Verification items for the finished model (mm, model axes). Face numbers are marked on the shaded views. A direction names the side the tool comes from. Coordinates: 2 decimals unless noted, no trailing zeros. Loops run counter-clockwise (first coordinate to the right, second up) from the corner with the lowest first, then second, coordinate; pieces in that order, holes last. Notation, with made-up numbers: (88.5, 77) -> (95.5, 77) arc R18 cw to (95.5, 90) -> close; hole circle Ø1 at (12.5, 53.5). An arc over 180 degrees is marked (long way). Answer as a JSON object with one key per item and string values. Group by question number.
Q1. Gauge pin test, flat ends, axial feed: pin 1 Ø2 at (x, z) = (2, -1) entering from +Y; pin 2 Ø1 at (x, y) = (7.5, 0.5) entering from +Z; pin 3 Ø1.5 at (x, y) = (12, -1.5) entering from +Z. Record the tip position at first contact, or that the pin passes through.
Q2. Cross-section at B-B on z = 0. Record the boundary of the cut face in (x, y), and give its area (3 significant figures).
Q3. Set-up check for the marked faces 1 and 2: record each of +Z, -Z, +X, -X, +Y, -Y from which the full face is reachable in a straight line by a thin tool's end or side.
Q4. Cross-section at A-A on y = 0. Record the boundary of the cut face in (x, z).
Q5. Scan lines: L1, parallel to X at y = -1.05, z = -1.3; L2, parallel to X at y = 1.7, z = 0; L3, parallel to Z at x = 7.5, y = 0.15. Record each from-to range of solid material in increasing order.
Q6. Cross-section at C-C on x = 5.5. Record the boundary of the cut face in (y, z), and give its area (3 significant figures).
```python
from build123d import *

# Parameters (mm, degrees)
CHAMFER1_SIZE       = 0.1
FILLET1_R           = 0.16
EXTRUDE1_DEPTH      = 15.059160715
EXTRUDE1_DEPTH_BACK = 15.059160715
SKETCH2_W           = 0.2
SKETCH2_H           = 0.2


with BuildPart() as part:
    # Sketch1 → Revolve1 (revolve)
    with BuildSketch(Plane.XY, mode=Mode.PRIVATE) as revolve1_sk:
        Polygon((0, 1.9), (0, 0), (13.8, 0), (13.8, 1), (1.3, 1), (1.3, 1.9), align=None)
    revolve(revolve1_sk.sketch.rotate(Axis((0, 0, 0), (1, 0, 0)), 90), axis=Axis((0, 0, 0), (1, 0, 0)))

    # Chamfer1
    chamfer1_edges = [part.edges().sort_by_distance(p)[0] for p in [
        (13.8, 0, -1),
    ]]
    chamfer(chamfer1_edges, length=CHAMFER1_SIZE)

    # Fillet1
    fillet1_edges = [part.edges().sort_by_distance(p)[0] for p in [
        (1.3, 0, -1),
    ]]
    fillet(fillet1_edges, radius=FILLET1_R)

    # Sketch2 → Extrude1 (cut, two sides: drawn at the far end of the back side and taken through both)
    with BuildSketch(Plane(origin=(0, 0, 0), x_dir=(1, 0, 0), z_dir=(0, 1, 0)).offset(-EXTRUDE1_DEPTH_BACK)):
        with Locations((0.1, -0.1)):
            Rectangle(SKETCH2_W, SKETCH2_H)
        with Locations((0.1, 0.1)):
            Rectangle(SKETCH2_W, SKETCH2_H)
    extrude(amount=EXTRUDE1_DEPTH + EXTRUDE1_DEPTH_BACK, mode=Mode.SUBTRACT)


solid = part.part
```
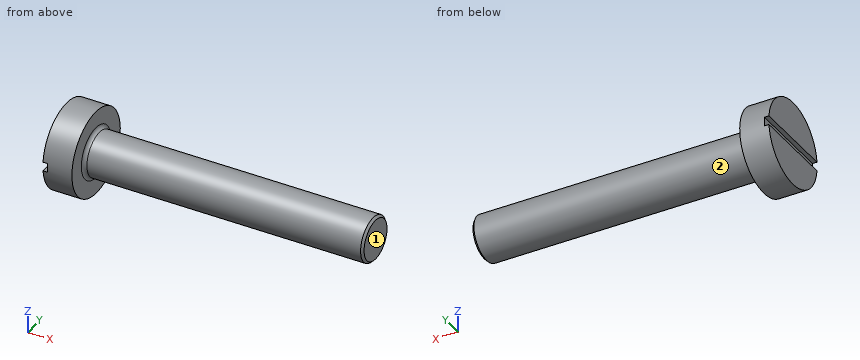
Computed values:
{
 "1": {"pin 1": "stops at y = 1.88", "pin 2": "stops at z = 1", "pin 3": "stops at z = 0.66"},
 "2": {"outline": "(0.2, -1.9) -> (1.3, -1.9) -> (1.3, -1.16) arc R0.16 cw to (1.46, -1) -> (13.7, -1) -> (13.8, -0.9) -> (13.8, 0.9) -> (13.7, 1) -> (1.46, 1) arc R0.16 cw to (1.3, 1.16) -> (1.3, 1.9) -> (0.2, 1.9) -> close", "area": "29.2 mm²"},
 "3": {"face 1": "+Z, -Z, +X, +Y, -Y", "face 2": "+X"},
 "4": {"outline": "(0, -1.9) -> (1.3, -1.9) -> (1.3, -1.16) arc R0.16 cw to (1.46, -1) -> (13.7, -1) -> (13.8, -0.9) -> (13.8, 0.9) -> (13.7, 1) -> (1.46, 1) arc R0.16 cw to (1.3, 1.16) -> (1.3, 1.9) -> (0, 1.9) -> (0, 0.2) -> (0.2, 0.2) -> (0.2, -0.2) -> (0, -0.2) -> close"},
 "5": {"L1": "x = 0 to 1.3", "L2": "x = 0.2 to 1.3", "L3": "z = -0.99 to 0.99"},
 "6": {"outline": "circle Ø2 at (0, 0)", "area": "3.14 mm²"}
}
